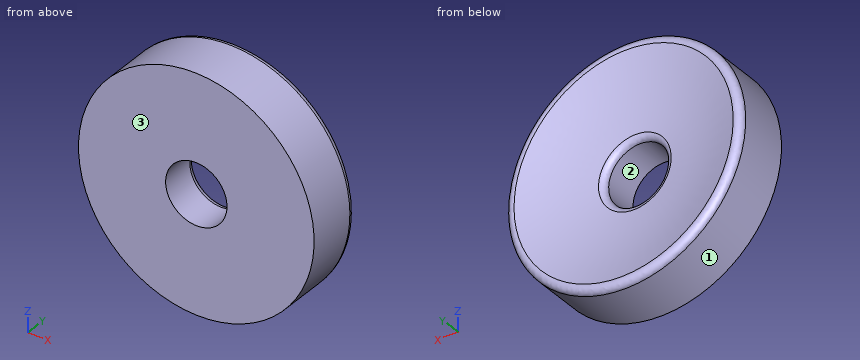
```python
from build123d import *

# Parameters (mm, degrees)
FILLET1_R = 1.016
FILLET2_R = 1.016


with BuildPart() as part:
    # Sketch1 → Revolve1 (revolve)
    with BuildSketch(Plane.XY, mode=Mode.PRIVATE) as revolve1_sk:
        with BuildLine():
            Line((4.9657, -63.283859201), (19.05, -63.283859201))
            Line((19.05, -63.283859201), (19.05, -53.881536726))
            ThreePointArc((19.05, -53.881536726), (12.104446693, -55.853423084), (4.9657, -56.933859201))
            Line((4.9657, -56.933859201), (4.9657, -63.283859201))
        make_face()
    revolve(revolve1_sk.sketch.rotate(Axis((0, 0, 0), (0, -1, 0)), 90), axis=Axis((0, 0, 0), (0, -1, 0)))  # turned: the seam where the file's is

    # Fillet1
    fillet1_edges = [part.edges().sort_by_distance(p)[0] for p in [
        (0, -53.881536726, -19.05),
    ]]
    fillet(fillet1_edges, radius=FILLET1_R)

    # Fillet2
    fillet2_edges = [part.edges().sort_by_distance(p)[0] for p in [
        (0, -56.933859201, -4.9657),
    ]]
    fillet(fillet2_edges, radius=FILLET2_R)


solid = part.part
```
Can you work these out from the model? Positions are in its coordinate system, mm. Face numbers are marked on the shaded views. Coordinates: 2 decimals unless noted, no trailing zeros. Loops run counter-clockwise (first coordinate to the right, second up) from the corner with the lowest first, then second, coordinate; pieces in that order, holes last. Notation, with made-up numbers: (32.5, 76.25) -> (74.5, 76.25) arc R25 cw to (74.5, 90.25) -> close; hole circle Ø11 at (-33, 36.25). An arc over 180 degrees is marked (long way). Put each result on its own line as item: value. Start each with the question number.
Q1. If I drill on line 1 (X direction, y = -59.9, z = 0); line 2 (X direction, y = -59, z = 3.5); line 3 (X direction, y = -61, z = 10), over which ranges is the centre line in solid material (lowest first)? Write a range as [from, to].
Q2. I want a section at A-A (y = -61.5). Write out the boundary of the cut face in (x, z), plus the area to 3 significant figures.
Q3. Thinking about a two-plate mould opening in X: for the marked faces 1, 2 and 3, which applies, pulls with the +X half, pulls with the -X half, needs draft (parallel to the pull), parting line crosses it, or undercut?
Q4. I'm going to push flat-ended pins straight in: P1, Ø4, axis at x = 12.5, y = -59.5, coming from the -Z side; P2, Ø4, axis at x = -13, y = -56, coming from the +Z side; P3, Ø1.5, axis at x = -10.5, z = -5, coming from the +Y side. Where does each tip first touch, or does it pass through?
Taken from the geometry:
1. line 1: x = [-19.05, -4.97], [4.97, 19.05]
1. line 2: x = [-18.73, -3.52], [3.52, 18.73]
1. line 3: x = [-16.21, 16.21]
2. outline: circle Ø38.1 at (0, 0); hole circle Ø9.93 at (0, 0)
2. area: 1,060 mm2
3. face 1: parting line crosses it
3. face 2: undercut
3. face 3: needs draft
4. P1: stops at z = -15.9
4. P2: stops at z = 15.55
4. P3: stops at y = -55.79
